```python
from build123d import *

# Parameters (mm, degrees)
F2_R      = 3.937
F2_R_2    = 2.667
F3_DEPTH  = 2.794
F4_R      = 5.08
F5_DEPTH  = 0.762
F6_R      = 7.239
F7_DEPTH  = 1.524
F9_R      = 11.049
F10_DEPTH = 1.524


with BuildPart() as f1:
    # F0 (on Right) → F1 (revolve)
    with BuildSketch(Plane.YZ):
        Polygon((2.4085466543, 2.8091624185), (2.4085466543, 0), (3.9751, 0), (3.937, 2.9743337072), (2.4085466543, 2.9743337072), align=None)
    revolve(axis=Axis((0, 0, 1.4871668536), (0, 0, 1)))



with BuildPart() as f3:
    # F2 (on Top) → F3 (new body)
    with BuildSketch(Plane.XY):
        Circle(F2_R)
        Circle(F2_R_2, mode=Mode.SUBTRACT)
    extrude(amount=F3_DEPTH)


with BuildPart() as f5:
    # F4 (on face) → F5 (new body)
    with BuildSketch(Plane(origin=(0, 0, 0), x_dir=(1, 0, 0), z_dir=(0, 0, -1))):
        Circle(F4_R)
    extrude(amount=F5_DEPTH)

    # F6 (on face) → F7 (join)
    with BuildSketch(Plane(origin=(0, 0, -0.762), x_dir=(1, 0, 0), z_dir=(0, 0, -1))):
        Circle(F6_R)
    extrude(amount=F7_DEPTH)


with BuildPart() as f1_1:
    add(f1.part)

    add(f5.part)  # F10 merges F5
    # F9 (on face) → F10 (join)
    with BuildSketch(Plane(origin=(0, 0, -2.286), x_dir=(1, 0, 0), z_dir=(0, 0, -1))):
        Circle(F9_R)
    extrude(amount=F10_DEPTH)


solid = f1_1.part
```
Geometry: final body of the model. Coordinates: model frame, mm. A direction names the side the tool comes from. Round coordinates to 2 decimals unless told otherwise and drop trailing zeros. Write each loop counter-clockwise with the first axis right and the second up, starting at its lowest first coordinate (ties: lowest second). Pieces come first, ordered by that corner, then holes.
Item 1: Set-up query: faces 1 (the face through (0, 0, -3.81)), 2 (the face through (2.3, 7.2, -2.286)). Return all of +Z, -Z, +X, -X, +Y, -Y with unobstructed straight access to the full face (end or side cutting, diameter ignored); none if empty.
Item 2: Section query C-C (z = 1.5). Return loops of the section in (x, y), plus the area to 3 significant figures.
Item 3: Section query B-B (z = -3). Return loops of the section in (x, y), plus the area to 3 significant figures.
Item 4: Pin query (flat end, axial travel): P1, Ø10, axis at x = 7.5, y = -7, coming from the +Z side; P2, Ø2, axis at x = 7, z = -1.5, coming from the -Y side; P3, Ø4, axis at x = 5.5, z = 0, coming from the -Y side. Return the tip coordinate at first contact, or that it passes through.
Item 5: Section query A-A (x = 5.5). Return loops of the section in (y, z), plus the area to 3 significant figures.
Item 6: Mould query, pull axis X, two halves, no side actions, for faces 3 (the face through (-0.661, -5.037, -0.376)), 4 (the face through (-3, 3, 0)), 5 (the face through (1.47, -1.91, 1.47)). Classes: +X half, -X half, draft (parallel to the pull), parting line (faces both ways), or undercut.
Item 7: Section query D-D (y = -9.25). Return loops of the section in (x, z), plus the area to 3 significant figures.
Item 8: Material intervals for L1, parallel to Z at x = 5.75, y = 4.75; L2, parallel to Z at x = 3, y = -3; L3, parallel to Y at x = 0, z = 1.6, sorted ascending.
Completed:
1. face 1: -Z, +X, -X, +Y, -Y
1. face 2: +Z
2. outline: circle Ø7.91 at (0, 0); hole circle Ø4.82 at (0, 0)
2. area: 30.9 mm2
3. outline: circle Ø22.1 at (0, 0)
3. area: 384 mm2
4. P1: stops at z = -0.76
4. P2: stops at y = -9.02
4. P3: stops at y = -6.25
5. outline: (-9.58, -3.81) - (9.58, -3.81) - (9.58, -2.29) - (4.71, -2.29) - (4.71, -0.76) - (-4.71, -0.76) - (-4.71, -2.29) - (-9.58, -2.29) - close
5. area: 43.6 mm2
6. face 3: parting line
6. face 4: draft
6. face 5: undercut
7. outline: (-6.04, -3.81) - (6.04, -3.81) - (6.04, -2.29) - (-6.04, -2.29) - close
7. area: 18.4 mm2
8. L1: z = -3.81 to -2.29
8. L2: z = -3.81 to 0
8. L3: y = -3.95 to -2.41, 2.41 to 3.95
